```python
from build123d import *

# Parameters (mm, degrees)
SKETCH3_R           = 3
CUT_EXTRUDE1_DEPTH  = 5
SKETCH4_W           = 2
SKETCH4_H           = 7.5
BOSS_EXTRUDE2_DEPTH = 10
SKETCH6_R           = 1.5
CUT_EXTRUDE2_DEPTH  = 10


with BuildPart() as part:
    # Sketch1 → Revolve2 (revolve)
    with BuildSketch(Plane.XY, mode=Mode.PRIVATE) as revolve2_sk:
        Polygon((0, 100), (10, 100), (10, 95), (7.75, 95), (7.75, 5), (10, 5), (10, 0), (0, 0), (0, 5), (5, 5), (5, 95), (0, 95), align=None)
    revolve(revolve2_sk.sketch.rotate(Axis((0, 100, 0), (0, -1, 0)), 180), axis=Axis((0, 100, 0), (0, -1, 0)))

    # Sketch3 → Cut-Extrude1 (cut)
    with BuildSketch(Plane(origin=(0, 100, 0), x_dir=(1, 0, 0), z_dir=(0, 1, 0))):
        with Locations(Location((0, 0, 0), (0, 0, 180))):
            Circle(SKETCH3_R)
    extrude(amount=-CUT_EXTRUDE1_DEPTH, mode=Mode.SUBTRACT)

    # Sketch4 → Boss-Extrude2 (add)
    with BuildSketch(Plane.XZ):
        with Locations((-2.5, 0)):
            Rectangle(SKETCH4_W, SKETCH4_H)
        with Locations((2.5, 0)):
            Rectangle(SKETCH4_W, SKETCH4_H)
    extrude(amount=BOSS_EXTRUDE2_DEPTH)

    # Sketch6 → Cut-Extrude2 (cut)
    with BuildSketch(Plane(origin=(3.5, 0, 0), x_dir=(0, 0, -1), z_dir=(1, 0, 0))):
        with Locations(Location((0, -7.5, 0), (0, 0, 90))):
            Circle(SKETCH6_R)
        with BuildLine():
            Line((-3.75, 0), (-2.75, -7.5))
            ThreePointArc((-2.75, -7.5), (0, -9.907670091), (2.75, -7.5))
            Line((2.75, -7.5), (3.75, 0))
            Line((3.75, 0), (3.75, -10))
            Line((3.75, -10), (-3.75, -10))
            Line((-3.75, -10), (-3.75, 0))
        make_face()
    extrude(amount=-CUT_EXTRUDE2_DEPTH, mode=Mode.SUBTRACT)


solid = part.part
```
Model file for the job. Use its own axes, mm. A direction names the side the tool comes from. Round coordinates to 2 decimals unless told otherwise and drop trailing zeros. Order: outer loops, then holes, each group sorted by start corner. A loop starts at its lowest first (then second) coordinate and runs counter-clockwise, first axis right, second up. Notation, with made-up numbers: M 84.5,-36.5 L 127.5,-36.5 A37 cw 127.5,-0.5 Z; hole C 64,-10.75 d11. An arc over 180 degrees is marked long. Use CSV: the item, a comma, the result in double quotes.
Item 1: Which spindle directions (+Z, -Z, +X, -X, +Y, -Y) get a long thin tool onto all of the face, cutting with end or side? Do faces 5 (the face through (-3.5, -4, 0)), 6 (the face through (-2.9, 95, 7.4)), 7 (the face through (1.5, -4, 0)), 8 (the face through (-2.486, -9.907, 0.056)), 9 (the face through (-2.486, -3.802, -3.243)). Say none if no direction does.
Worked answers:
face 5,"+Z, -Z, -X, -Y"
face 6,"none"
face 7,"+Z, -Z, -Y"
face 8,"+X, -X, -Y"
face 9,"-Z, +X, -X, -Y"
Item 2: Pull direction Y, two halves, no side cores. Call faces 1 (the face through (-2.86, 97.54, 0.9)), 2 (the face through (2.514, -3.698, 3.257)), 3 (the face through (2.9, 5, 7.4)), 4 (the face through (2.1, 100, -2.4)): released by +Y, released by -Y, zero draft, split by the parting line, or undercut.
Worked answers:
face 1,"zero draft"
face 2,"released by -Y"
face 3,"undercut"
face 4,"released by +Y"
Item 3: Saw through at A-A (x = 0). List the corners of the cut face in (y, z).
Worked answers:
outline,"M 0,-10 L 5,-10 L 5,-7.75 L 95,-7.75 L 95,-10 L 100,-10 L 100,-3 L 95,-3 L 95,-5 L 5,-5 L 5,5 L 95,5 L 95,3 L 100,3 L 100,10 L 95,10 L 95,7.75 L 5,7.75 L 5,10 L 0,10 Z"
Item 4: Saw through at C-C (x = 8.75). List the corners of the cut face in (y, z).
Worked answers:
outline,"M 0,-4.84 L 5,-4.84 L 5,4.84 L 0,4.84 Z; M 95,-4.84 L 100,-4.84 L 100,4.84 L 95,4.84 Z"
Item 5: Saw through at D-D (y = 30.5). List the corners of the cut face in (x, z), plus the area to 3 significant figures.
Worked answers:
outline,"C 0,0 d15.5; hole C 0,0 d10"
area,"110 mm²"
Item 6: Saw through at B-B (z = 0). State how many separate pieces and enclosed holes the cut face has, plus the area to 3 significant figures.
Worked answers:
separate pieces,"3"
enclosed holes,"0"
area,"693 mm²"
Item 7: Probe probe 1 along Y at (x, z) = (4.25, -8.25); probe 2 along Z at (x, y) = (0, 98.6); probe 3 along X at (y, z) = (-0.5, 2.75). List the from-to ranges inside material, lowest first.
Worked answers:
probe 1,"0 to 5, 95 to 100"
probe 2,"-10 to -3, 3 to 10"
probe 3,"-3.5 to -1.5, 1.5 to 3.5"
Item 8: Pin check, flat tips, straight feed: pin 1 (2 mm diameter, centred on y = -7, z = 0.5, fed in from +X); pin 2 (1.5 mm diameter, centred on x = 0, z = -3, fed in from -Y); pin 3 (5 mm diameter, centred on y = 41, z = -6.5, fed in from -X); pin 4 (1.8 mm diameter, centred on y = -7.5, z = 0, fed in from +X). Stop position of each tip, or through.
Worked answers:
pin 1,"x = 3.5"
pin 2,"y = 0"
pin 3,"x = -6.64"
pin 4,"through"
